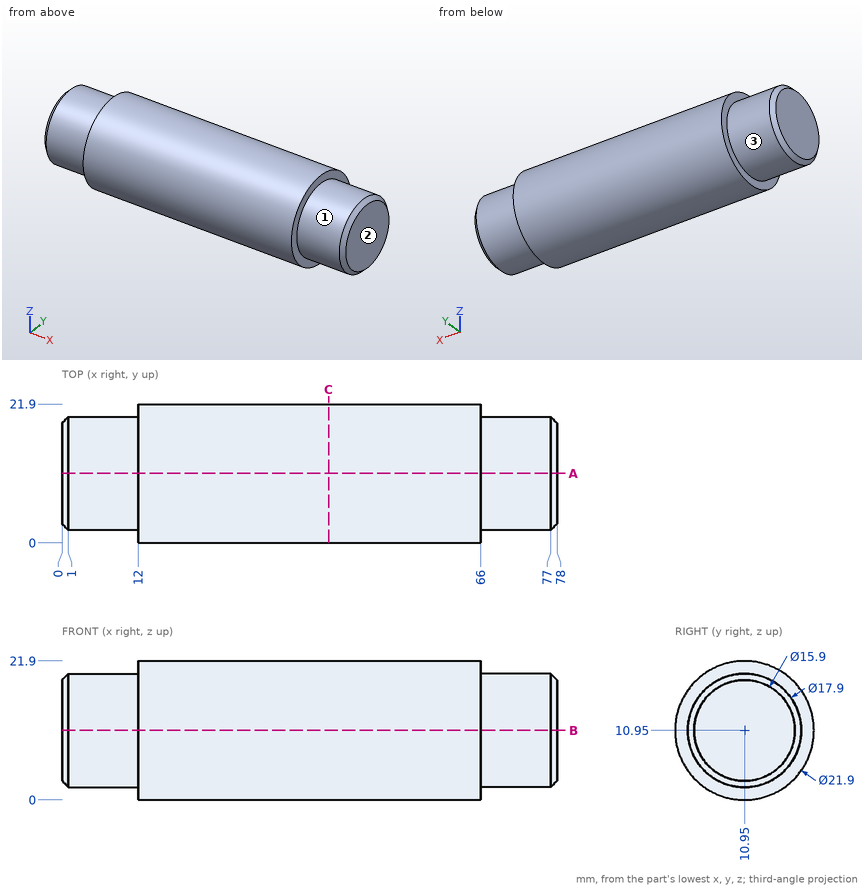
Drawing for the job (mm, zero at the part's lowest x, y, z). A direction names the side the tool comes from. Round coordinates to 2 decimals unless told otherwise and drop trailing zeros. Order: outer loops, then holes, each group sorted by start corner. A loop starts at its lowest first (then second) coordinate and runs counter-clockwise, first axis right, second up.
Item 1: Probe line 1 along X through (y, z) = (4.5, 17.5); line 2 along Y through (x, z) = (59.5, 11.5); line 3 along Y through (x, z) = (38, 5.5). List the from-to ranges inside material, lowest first.
Item 2: Saw through at C-C on x = 42. Write the cut outline in (y, z), then the cut area to 3 significant figures.
Item 3: Tool access for the marked faces 1, 2 and 3: list every direction of +Z, -Z, +X, -X, +Y, -Y with a clear straight run to the whole face (end or side of a thin tool).
Item 4: Saw through at A-A on y = 10.95. Write the cut outline in (x, z).
Item 5: Pin check, flat tips, straight feed: pin 1 (4 mm diameter, centred on x = 62, y = 16, fed in from +Z); pin 2 (2 mm diameter, centred on x = 21, z = 4.5, fed in from -Y); pin 3 (1 mm diameter, centred on x = 49, y = 12.5, fed in from +Z). Stop position of each tip, or through.
Reported:
1. line 1: x = 12 to 66
1. line 2: y = 0.01 to 21.89
1. line 3: y = 1.45 to 20.45
2. outline: circle Ø21.9 at (10.95, 10.95)
2. area: 377 mm2
3. face 1: +X
3. face 2: +Z, -Z, +X, +Y, -Y
3. face 3: -X
4. outline: (0, 3) - (1, 2) - (12, 2) - (12, 0) - (66, 0) - (66, 2) - (77, 2) - (78, 3) - (78, 18.9) - (77, 19.9) - (66, 19.9) - (66, 21.9) - (12, 21.9) - (12, 19.9) - (1, 19.9) - (0, 18.9) - close
5. pin 1: stops at z = 21.47
5. pin 2: stops at y = 1.45
5. pin 3: stops at z = 21.85
